Could you check a few things on this model? Use its own coordinates, in mm. Face numbers are marked on the shaded views. Round coordinates to 2 decimals unless told otherwise and drop trailing zeros. Write each loop counter-clockwise with the first axis right and the second up, starting at its lowest first coordinate (ties: lowest second). Pieces come first, ordered by that corner, then holes. Notation, with made-up numbers: M -25,-9.75 L 14,-9.75 A35 ccw 14,29.25 Z; hole C 32.25,8 d9. An arc over 180 degrees is marked long. One line per item, written item: value. Start each with the question number.
(1) I want a section at D-D on y = 40.75. Please give me the cut outline in (x, z), and give its area (3 significant figures).
(2) I want a section at B-B on x = 0. Please give me the cut outline in (y, z).
(3) Thinking about a two-plate mould opening in Z: for the marked faces 1, 2 and 3, which applies, released by +Z, released by -Z, zero draft, split by the parting line, or undercut?
(4) If I drill on L1, parallel to X at y = 25, z = -19; L2, parallel to Z at x = 0, y = 45; L3, parallel to Z at x = -17.5, y = 29, over which ranges is the centre line in solid material (lowest first)?
(5) I'm going to push flat-ended pins straight in: pin 1 Ø10 at (x, z) = (11.5, 10.5) entering from +Y; pin 2 Ø8 at (x, y) = (20, 43) entering from +Z; pin 3 Ø12 at (x, z) = (-9, -1.5) entering from +Y. Where does each tip first touch, or does it pass through?
(6) I want a section at C-C on y = 33.5. Please give me the cut outline in (x, z), and give its area (3 significant figures).
(7) I want a section at A-A on z = 0. Please give me the cut outline in (x, y).
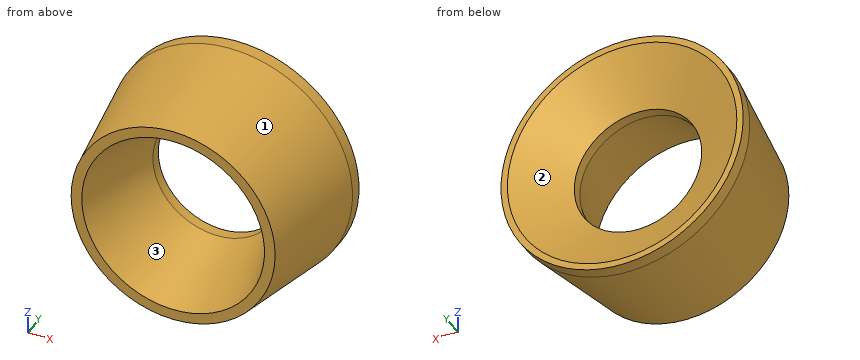
Autodesk Inventor part; units mm, degrees
ref_plane "YZ Plane" through (0, 0, 0) normal (1, 0, 0) x (0, 1, 0)
ref_plane "XZ Plane" through (0, 0, 0) normal (0, 1, 0) x (-1, 0, 0)
ref_plane "XY Plane" through (0, 0, 0) normal (0, 0, 1) x (1, 0, 0)
sketch "Boceto1" plane through (0, 0, 0) normal (0, 0, 1) x (1, 0, 0)
  line L0 (-24, 23.6746) -> (-21.5, 23.6746)
  line L1 (-28.5, 50.5) -> (-24, 23.6746)
  line L2 (-28.5, 50.5) -> (-28.5, 53.5)
  line L3 (-28.5, 53.5) -> (-27, 53.5)
  line L4 (-27, 53.5) -> (-15, 46.1746)
  line L5 (-15, 46.1746) -> (-15, 43.6746)
  line L6 (-15, 43.6746) -> (-21.5, 23.6746)
  line L7 (0, -10.7) -> (0, 64.2)
  point P0 (0, 0)
  dimension "d5" = 2.5
  dimension "d6" = 4.5
  dimension "d7" = 3
  dimension "d8" = 1.5
  dimension "d9" = 12
  dimension "d10" = 2.5
  dimension "d11" = 20
revolve "Revolución1" add sketch "Boceto1" angle 360 about axis through (0, -10, 0) along (0, 1, 0)
properties part number "GRAFITO"
Found:
1. outline: C 0,0 d53.73; hole C 0,0 d31.9
1. area: 1,470 mm²
2. outline: M 23.67,-24 L 50.5,-28.5 L 53.5,-28.5 L 53.5,-27 L 46.17,-15 L 43.67,-15 L 23.67,-21.5 Z; M 23.67,21.5 L 43.67,15 L 46.17,15 L 53.5,27 L 53.5,28.5 L 50.5,28.5 L 23.67,24 Z
3. face 1: split by the parting line
3. face 2: undercut
3. face 3: undercut
4. L1: x = -15.02 to -9.11, 9.11 to 15.02
4. L2: z = -27.58 to -15, 15 to 27.58
4. L3: z = -17.7 to -9.2, 9.2 to 17.7
5. pin 1: stops at y = 49.58
5. pin 2: stops at z = 22.16
5. pin 3: stops at y = 46.25
6. outline: C 0,0 d51.3; hole C 0,0 d36.61
6. area: 1,010 mm²
7. outline: M -28.5,50.5 L -24,23.67 L -21.5,23.67 L -15,43.67 L -15,46.17 L -27,53.5 L -28.5,53.5 Z; M 15,43.67 L 21.5,23.67 L 24,23.67 L 28.5,50.5 L 28.5,53.5 L 27,53.5 L 15,46.17 Z
